Part model, mm, in its own coordinate system. Face numbers are marked on the shaded views. A direction names the side the tool comes from. Give positions to 0.01 mm unless a question says otherwise; leave off trailing zeros. Order: outer loops, then holes, each group sorted by start corner. A loop starts at its lowest first (then second) coordinate and runs counter-clockwise, first axis right, second up.
1. Slice it at A-A on x = 0. List the corners of the cut face in (y, z).
2. Slice it at D-D on x = -22.5. List the corners of the cut face in (y, z), and give its area (3 significant figures).
3. Probe line 1 (Y direction, x = 27, z = 6.5); line 2 (Y direction, x = 0, z = 57.5); line 3 (Z direction, x = -18, y = 28). List the from-to ranges inside material, lowest first.
4. Which spindle directions (+Z, -Z, +X, -X, +Y, -Y) get a long thin tool onto all of the face, cutting with end or side? Do the marked faces 1, 2 and 3. Say none if no direction does.
5. Mould opens along Z. For the marked faces 4, 5 and 6 say: +Z half, -Z half, draft (parallel to the pull), parting line (faces both ways), or undercut.
6. Drop flat-ended pins along their axis: pin 1 Ø9 at (x, y) = (27, -27) entering from -Z; pin 2 Ø8 at (x, z) = (-26.5, 34) entering from +Y; pin 3 Ø7 at (x, y) = (0, 28) entering from +Z; pin 4 Ø4 at (y, z) = (-4.5, 45.5) entering from -X. Give the stop position or say it passes through.
7. Slice it at C-C on z = 55. List the corners of the cut face in (x, y).
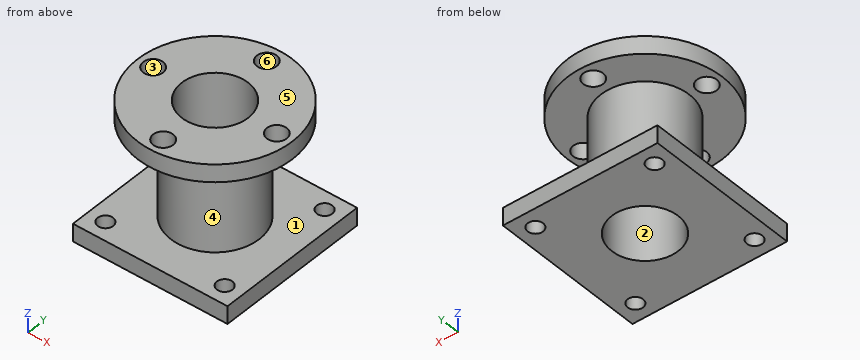
from build123d import *

# Parameters (mm, degrees)
SKETCH_1_R          = 20
EXTRUDE_1_DEPTH     = 60
SKETCH_2_W          = 70
SKETCH_2_H          = 70
EXTRUDE_2_DEPTH     = 8
SKETCH_3_R          = 35
EXTRUDE_3_DEPTH     = 8
SKETCH_4_R          = 15
CUT_EXTRUDE_1_DEPTH = 71
SKETCH_5_R          = 3.5
CUT_EXTRUDE_2_DEPTH = 8
SKETCH_6_R          = 4.5
CUT_EXTRUDE_3_DEPTH = 8


with BuildPart() as part:
    # 草图1 → 凸台-拉伸1 (new body)
    with BuildSketch(Plane.XY):
        Circle(SKETCH_1_R)
    extrude(amount=EXTRUDE_1_DEPTH)

    # 草图2 → 凸台-拉伸2 (add)
    with BuildSketch(Plane.XY):
        Rectangle(SKETCH_2_W, SKETCH_2_H)
    extrude(amount=EXTRUDE_2_DEPTH)

    # 草图3 → 凸台-拉伸3 (add)
    with BuildSketch(Plane.XY.offset(52)):
        Circle(SKETCH_3_R)
    extrude(amount=EXTRUDE_3_DEPTH)

    # 草图4 → 切除-拉伸1 (cut, symmetric)
    with BuildSketch(Plane.XY):
        Circle(SKETCH_4_R)
    extrude(amount=CUT_EXTRUDE_1_DEPTH, both=True, mode=Mode.SUBTRACT)

    # 草图5 → 切除-拉伸2 (cut)
    with BuildSketch(Plane.XY):
        with Locations((27, 27)):
            Circle(SKETCH_5_R)
        with Locations((-27, 27)):
            Circle(SKETCH_5_R)
        with Locations((-27, -27)):
            Circle(SKETCH_5_R)
        with Locations((27, -27)):
            Circle(SKETCH_5_R)
    extrude(amount=CUT_EXTRUDE_2_DEPTH, mode=Mode.SUBTRACT)

    # 草图6 → 切除-拉伸3 (cut)
    with BuildSketch(Plane.XY.offset(60)):
        with Locations((28, 0)):
            Circle(SKETCH_6_R)
        with Locations((0, 28)):
            Circle(SKETCH_6_R)
        with Locations((-28, 0)):
            Circle(SKETCH_6_R)
        with Locations((0, -28)):
            Circle(SKETCH_6_R)
    extrude(amount=-CUT_EXTRUDE_3_DEPTH, mode=Mode.SUBTRACT)


solid = part.part
Data:
1. outline: (-35, 0) - (-15, 0) - (-15, 60) - (-23.5, 60) - (-23.5, 52) - (-20, 52) - (-20, 8) - (-35, 8) - close; (-35, 52) - (-32.5, 52) - (-32.5, 60) - (-35, 60) - close; (15, 0) - (35, 0) - (35, 8) - (20, 8) - (20, 52) - (23.5, 52) - (23.5, 60) - (15, 60) - close; (32.5, 52) - (35, 52) - (35, 60) - (32.5, 60) - close
2. outline: (-35, 0) - (35, 0) - (35, 8) - (-35, 8) - close; (-26.81, 52) - (26.81, 52) - (26.81, 60) - (-26.81, 60) - close
2. area: 989 mm2
3. line 1: y = -35 to -30.5, -23.5 to 23.5, 30.5 to 35
3. line 2: y = -35 to -32.5, -23.5 to -15, 15 to 23.5, 32.5 to 35
3. line 3: z = 0 to 8, 52 to 60
4. face 1: none
4. face 2: +Z, -Z
4. face 3: +Z
5. face 4: undercut
5. face 5: +Z half
5. face 6: draft
6. pin 1: stops at z = 0
6. pin 2: passes through
6. pin 3: stops at z = 8
6. pin 4: stops at x = -19.84
7. outline: circle Ø70 at (0, 0); hole circle Ø9 at (-28, 0); hole circle Ø30 at (0, 0); hole circle Ø9 at (0, -28); hole circle Ø9 at (0, 28); hole circle Ø9 at (28, 0)
